from build123d import *

# Parameters (mm, degrees)
SKETCH1_W           = 100
SKETCH1_H           = 100
SKETCH1_R           = 1.6
SKETCH1_W_2         = 3
SKETCH1_H_2         = 1.3
SKETCH1_W_3         = 1.3
SKETCH1_H_3         = 3
BOSS_EXTRUDE1_DEPTH = 8


with BuildPart() as part:
    # Sketch1 → Boss-Extrude1 (new body)
    with BuildSketch(Plane(origin=(0, 0, 0), x_dir=(1, 0, 0), z_dir=(0, 1, 0))):
        Rectangle(SKETCH1_W, SKETCH1_H)
        with Locations(Location((26.5, 28.7, 0), (0, 0, 270))):
            Circle(SKETCH1_R, mode=Mode.SUBTRACT)
        with Locations(Location((-10.7, 30.2, 0), (0, 0, 270))):
            Circle(SKETCH1_R, mode=Mode.SUBTRACT)
        with Locations((19, -14.35)):
            Rectangle(SKETCH1_W_2, SKETCH1_H_2, mode=Mode.SUBTRACT)
        with Locations((-4, -14.35)):
            Rectangle(SKETCH1_W_2, SKETCH1_H_2, mode=Mode.SUBTRACT)
        with Locations((-15.65, -28.25)):
            Rectangle(SKETCH1_W_3, SKETCH1_H_3, mode=Mode.SUBTRACT)
        with Locations((30.65, -28.25)):
            Rectangle(SKETCH1_W_3, SKETCH1_H_3, mode=Mode.SUBTRACT)
        with Locations((19, -42.15)):
            Rectangle(SKETCH1_W_2, SKETCH1_H_2, mode=Mode.SUBTRACT)
        with Locations((-4, -42.15)):
            Rectangle(SKETCH1_W_2, SKETCH1_H_2, mode=Mode.SUBTRACT)
    extrude(amount=BOSS_EXTRUDE1_DEPTH)


solid = part.part
Here's how the part is built. I have some questions about the finished solid (model axes, mm). A direction names the side the tool comes from. Give positions to 0.01 mm unless a question says otherwise; leave off trailing zeros. Order: outer loops, then holes, each group sorted by start corner. A loop starts at its lowest first (then second) coordinate and runs counter-clockwise, first axis right, second up. Notation, with made-up numbers: (2, -25.75) -> (29, -25.75) arc R20 ccw to (29, 7.25) -> close; hole circle Ø8 at (41, 26). An arc over 180 degrees is marked (long way). Use a Markdown table: item, result. Add a question column.
Item 1: If we mould it in two halves opening along Z, with no side actions, what happens to faces 1 (the face through (-15, 4, 28)), 2 (the face through (50, 4, 1)), 3 (the face through (-1, 4, -50))? For each: pulls with the +Z half, pulls with the -Z half, needs draft (parallel to the pull), parting line crosses it, or undercut.
Item 2: Imagine slicing it at A-A on x = -4. Please give me the cut outline in (y, z).
Item 3: For faces 4 (the face through (-4, 4, 41.5)), 5 (the face through (-1, 4, 50)), which set-ups out of +Z, -Z, +X, -X, +Y, -Y let a thin tool reach every point of the face, with its end or its side?
Data:
| question | item | result |
|---|---|---|
| 1 | face 1 | undercut |
| 1 | face 2 | needs draft |
| 1 | face 3 | pulls with the -Z half |
| 2 | outline | (0, -50) -> (8, -50) -> (8, 13.7) -> (0, 13.7) -> close; (0, 15) -> (8, 15) -> (8, 41.5) -> (0, 41.5) -> close; (0, 42.8) -> (8, 42.8) -> (8, 50) -> (0, 50) -> close |
| 3 | face 4 | +Y, -Y |
| 3 | face 5 | +Z, +X, -X, +Y, -Y |
